Input: part model. Units: mm. Frame: model coordinates. Coordinates: 2 decimals unless noted, no trailing zeros. Order: outer loops, then holes, each group sorted by start corner. A loop starts at its lowest first (then second) coordinate and runs counter-clockwise, first axis right, second up. Notation, with made-up numbers: (21.25, 38) - (30.25, 38) arc R27 cw to (30.25, 71) - close; hole circle Ø1 at (78.25, -3.5). An arc over 180 degrees is marked (long way). Use a Markdown table: item, result. Add a question column.
from build123d import *

# Parameters (mm, degrees)
F0_W     = 150
F0_H     = 150
F0_W_2   = 6.1
F0_H_2   = 6.1
F1_DEPTH = 25


with BuildPart() as f1:
    # F0 (on Top) → F1 (new body)
    with BuildSketch(Plane.XY):
        with Locations((-18.306946, 1.062334)):
            Rectangle(F0_W, F0_H)
        with Locations((-73.323034, -50.083685)):
            Rectangle(F0_W_2, F0_H_2, mode=Mode.SUBTRACT)
        with Locations((-55.023034, -50.083685)):
            Rectangle(F0_W_2, F0_H_2, mode=Mode.SUBTRACT)
        with Locations((-36.723034, -50.083685)):
            Rectangle(F0_W_2, F0_H_2, mode=Mode.SUBTRACT)
        with Locations((-18.423034, -50.083685)):
            Rectangle(F0_W_2, F0_H_2, mode=Mode.SUBTRACT)
        with Locations((-73.323034, -24.783685)):
            Rectangle(F0_W_2, F0_H_2, mode=Mode.SUBTRACT)
        with Locations((-73.323034, 0.516315)):
            Rectangle(F0_W_2, F0_H_2, mode=Mode.SUBTRACT)
        with Locations((-55.023034, -24.783685)):
            Rectangle(F0_W_2, F0_H_2, mode=Mode.SUBTRACT)
        with Locations((-36.723034, -24.783685)):
            Rectangle(F0_W_2, F0_H_2, mode=Mode.SUBTRACT)
        with Locations((-18.423034, -24.783685)):
            Rectangle(F0_W_2, F0_H_2, mode=Mode.SUBTRACT)
        with Locations((-55.023034, 0.516315)):
            Rectangle(F0_W_2, F0_H_2, mode=Mode.SUBTRACT)
        with Locations((-36.723034, 0.516315)):
            Rectangle(F0_W_2, F0_H_2, mode=Mode.SUBTRACT)
        with Locations((-18.423034, 0.516315)):
            Rectangle(F0_W_2, F0_H_2, mode=Mode.SUBTRACT)
        with Locations((-0.123034, -50.083685)):
            Rectangle(F0_W_2, F0_H_2, mode=Mode.SUBTRACT)
        with Locations((18.176966, -50.083685)):
            Rectangle(F0_W_2, F0_H_2, mode=Mode.SUBTRACT)
        with Locations((36.476966, -50.083685)):
            Rectangle(F0_W_2, F0_H_2, mode=Mode.SUBTRACT)
        with Locations((-0.123034, -24.783685)):
            Rectangle(F0_W_2, F0_H_2, mode=Mode.SUBTRACT)
        with Locations((18.176966, -24.783685)):
            Rectangle(F0_W_2, F0_H_2, mode=Mode.SUBTRACT)
        with Locations((-0.123034, 0.516315)):
            Rectangle(F0_W_2, F0_H_2, mode=Mode.SUBTRACT)
        with Locations((18.176966, 0.516315)):
            Rectangle(F0_W_2, F0_H_2, mode=Mode.SUBTRACT)
        with Locations((36.476966, -24.783685)):
            Rectangle(F0_W_2, F0_H_2, mode=Mode.SUBTRACT)
        with Locations((36.476966, 0.516315)):
            Rectangle(F0_W_2, F0_H_2, mode=Mode.SUBTRACT)
        with Locations((-73.323034, 25.816315)):
            Rectangle(F0_W_2, F0_H_2, mode=Mode.SUBTRACT)
        with Locations((-55.023034, 25.816315)):
            Rectangle(F0_W_2, F0_H_2, mode=Mode.SUBTRACT)
        with Locations((-36.723034, 25.816315)):
            Rectangle(F0_W_2, F0_H_2, mode=Mode.SUBTRACT)
        with Locations((-18.423034, 25.816315)):
            Rectangle(F0_W_2, F0_H_2, mode=Mode.SUBTRACT)
        with Locations((-73.323034, 51.116315)):
            Rectangle(F0_W_2, F0_H_2, mode=Mode.SUBTRACT)
        with Locations((-55.023034, 51.116315)):
            Rectangle(F0_W_2, F0_H_2, mode=Mode.SUBTRACT)
        with Locations((-36.723034, 51.116315)):
            Rectangle(F0_W_2, F0_H_2, mode=Mode.SUBTRACT)
        with Locations((-18.423034, 51.116315)):
            Rectangle(F0_W_2, F0_H_2, mode=Mode.SUBTRACT)
        with Locations((-0.123034, 25.816315)):
            Rectangle(F0_W_2, F0_H_2, mode=Mode.SUBTRACT)
        with Locations((18.176966, 25.816315)):
            Rectangle(F0_W_2, F0_H_2, mode=Mode.SUBTRACT)
        with Locations((36.476966, 25.816315)):
            Rectangle(F0_W_2, F0_H_2, mode=Mode.SUBTRACT)
        with Locations((-0.123034, 51.116315)):
            Rectangle(F0_W_2, F0_H_2, mode=Mode.SUBTRACT)
        with Locations((18.176966, 51.116315)):
            Rectangle(F0_W_2, F0_H_2, mode=Mode.SUBTRACT)
        with Locations((36.476966, 51.116315)):
            Rectangle(F0_W_2, F0_H_2, mode=Mode.SUBTRACT)
    extrude(amount=F1_DEPTH)


solid = f1.part
1) Material intervals for L1, parallel to Y at x = -17, z = 22, sorted ascending.
2) Pull-direction query (Y, two-part tool) for faces 1 (the flat face through (56.693, 0, 12)), 2 (the flat face through (-73, 3.566, 12)), 3 (the flat face through (-19, 76.062, 12)), 4 (the flat face through (2.927, 51, 12)); classes: pulls with the +Y half, pulls with the -Y half, needs draft (parallel to the pull), parting line crosses it, or undercut.
3) Cut plane A-A (x = -18). Return the cut outline in (y, z).
4) Contact query for a flat-ended pin moving along its axis: P1, Ø10, axis at x = -10.5, y = -8.5, coming from the -Z side. Output: stop coordinate, or through.
5) Cut plane B-B (z = 13). State how many separate pieces and enclosed holes the cut face has, and give its area (3 significant figures).
Computed:
| question | item | result |
|---|---|---|
| 1 | L1 | y = -73.94 to -53.13, -47.03 to -27.83, -21.73 to -2.53, 3.57 to 22.77, 28.87 to 48.07, 54.17 to 76.06 |
| 2 | face 1 | needs draft |
| 2 | face 2 | undercut |
| 2 | face 3 | pulls with the +Y half |
| 2 | face 4 | undercut |
| 3 | outline | (-73.94, 0) - (-53.13, 0) - (-53.13, 25) - (-73.94, 25) - close; (-47.03, 0) - (-27.83, 0) - (-27.83, 25) - (-47.03, 25) - close; (-21.73, 0) - (-2.53, 0) - (-2.53, 25) - (-21.73, 25) - close; (3.57, 0) - (22.77, 0) - (22.77, 25) - (3.57, 25) - close; (28.87, 0) - (48.07, 0) - (48.07, 25) - (28.87, 25) - close; (54.17, 0) - (76.06, 0) - (76.06, 25) - (54.17, 25) - close |
| 4 | P1 | stops at z = 0 |
| 5 | separate pieces | 1 |
| 5 | enclosed holes | 35 |
| 5 | area | 21,200 mm2 |
